Build history of the part. All positions in model axes, mm. A direction names the side the tool comes from. Coordinates: 2 decimals unless noted, no trailing zeros. Loops run counter-clockwise (first coordinate to the right, second up) from the corner with the lowest first, then second, coordinate; pieces in that order, holes last. Notation, with made-up numbers: (-12.5, 17) - (13.5, 17) arc R23 ccw to (13.5, 38) - close; hole circle Ø5 at (40, 2). An arc over 180 degrees is marked (long way). One line per item, written item: value.
```python
from build123d import *

# Parameters (mm, degrees)
BOTTOM_SECTION_BASE_SKETCH_W             = 15
BOTTOM_SECTION_BASE_SKETCH_H             = 15
BOTTOM_SECTION_EXTRUDE_DEPTH             = 40
HINGE_CUTOUT_SKETCH_W                    = 7
HINGE_CUTOUT_SKETCH_H                    = 15
HINGE_CUTOUT_EXTRUDED_CUT_DEPTH          = 15
HINGE_HOLE_SKETCH_R                      = 1
HINGE_HOLE_EXTRUDED_CUT_DEPTH            = 44.373378932
HINGER_CORNER_FILLETS_R                  = 5
STYLE_FILLETS_R                          = 1
ROUTING_HOLES_SKETCH_W                   = 2
ROUTING_HOLES_SKETCH_H                   = 2
ROUTING_HOLES_EXTRUDED_CUT_DEPTH         = 42.382363393
BACKING_START                            = -3.5
BACKING_EXTRUDE_DEPTH                    = 7
BOTTOM_SECTION_CONNECTION_HOLE_R         = 1.75
BOTTOM_SECTION_CONNECTION_HOLE_CUT_DEPTH = 3
SKETCH2_W                                = 7
SKETCH2_H                                = 2
BOTTOM_EXTENSION_EXTRUDE_DEPTH           = 6.5
FILLET1_R                                = 0.5


# Read off the part's stored shape, not the designer's step: Backing Extrude
with BuildPart() as part:
    # Bottom Section Base Sketch → Bottom Section Extrude (new body)
    with BuildSketch(Plane.XY):
        Rectangle(BOTTOM_SECTION_BASE_SKETCH_W, BOTTOM_SECTION_BASE_SKETCH_H)
    extrude(amount=BOTTOM_SECTION_EXTRUDE_DEPTH)

    # Hinge Cutout Sketch → Hinge Cutout Extruded Cut (cut)
    with BuildSketch(Plane.XY):
        Rectangle(HINGE_CUTOUT_SKETCH_W, HINGE_CUTOUT_SKETCH_H)
    hinge_cutout_extruded_cut = extrude(amount=HINGE_CUTOUT_EXTRUDED_CUT_DEPTH, mode=Mode.SUBTRACT)

    # Hinge Hole Sketch → Hinge Hole Extruded Cut (cut, through all)
    with BuildSketch(Plane(origin=(7.5, 0, 0), x_dir=(0, 0, -1), z_dir=(1, 0, 0))):
        with Locations((-5, 0)):
            Circle(HINGE_HOLE_SKETCH_R)
    hinge_hole_extruded_cut = extrude(amount=-HINGE_HOLE_EXTRUDED_CUT_DEPTH, mode=Mode.SUBTRACT)

    # Hinge and Hole Cutout Mirror: Hinge Cutout Extruded Cut, Hinge Hole Extruded Cut across plane
    add(hinge_cutout_extruded_cut.mirror(Plane.XY.offset(20)), mode=Mode.SUBTRACT)
    add(hinge_hole_extruded_cut.mirror(Plane.XY.offset(20)), mode=Mode.SUBTRACT)

    # Hinger Corner Fillets
    hinger_corner_fillets_edges = [part.edges().sort_by_distance(p)[0] for p in [
        (5.5, -7.5, 0),
        (-5.5, 7.5, 0),
        (-5.5, -7.5, 40),
        (-5.5, 7.5, 40),
        (5.5, -7.5, 40),
        (-5.5, -7.5, 0),
        (5.5, 7.5, 0),
        (5.5, 7.5, 40),
    ]]
    fillet(hinger_corner_fillets_edges, radius=HINGER_CORNER_FILLETS_R)

    # Style Fillets
    style_fillets_edges = [part.edges().sort_by_distance(p)[0] for p in [
        (7.5, 0, 40),
        (7.5, 7.5, 20),
        (-7.5, 7.5, 20),
        (7.5, 0, 0),
        (7.5, -7.5, 20),
        (7.5, 6.035533906, 1.464466094),
        (7.5, -6.035533906, 1.464466094),
        (7.5, -6.035533906, 38.535533906),
        (7.5, 6.035533906, 38.535533906),
        (-7.5, -7.5, 20),
        (-7.5, 0, 40),
        (-7.5, 0, 0),
        (-7.5, -6.035533906, 1.464466094),
        (-7.5, 6.035533906, 1.464466094),
        (-7.5, 6.035533906, 38.535533906),
        (-7.5, -6.035533906, 38.535533906),
    ]]
    fillet(style_fillets_edges, radius=STYLE_FILLETS_R)

    # Routing Holes Sketch → Routing Holes Extruded Cut (cut, through all)
    with BuildSketch(Plane.XY):
        with Locations((0, 4.5)):
            Rectangle(ROUTING_HOLES_SKETCH_W, ROUTING_HOLES_SKETCH_H)
        with Locations((0, -4.5)):
            Rectangle(ROUTING_HOLES_SKETCH_W, ROUTING_HOLES_SKETCH_H)
    extrude(amount=ROUTING_HOLES_EXTRUDED_CUT_DEPTH, mode=Mode.SUBTRACT)

    # Backing Extrude outline → Backing Extrude (add)
    with BuildSketch(Plane.YZ.offset(BACKING_START)):
        Polygon((-7.5, 32.145884327), (-7.5, 25), (-5.5, 25), (-5.5, 32.106829325), align=None)
    extrude(amount=BACKING_EXTRUDE_DEPTH)

    # Bottom Section Connection Hole → Bottom Section Connection Hole Cut (cut)
    with BuildSketch(Plane(origin=(7.5, 0, 0), x_dir=(0, 0, -1), z_dir=(1, 0, 0))):
        with Locations((-20, 0)):
            Circle(BOTTOM_SECTION_CONNECTION_HOLE_R)
    bottom_section_connection_hole_cut = extrude(amount=-BOTTOM_SECTION_CONNECTION_HOLE_CUT_DEPTH, mode=Mode.SUBTRACT)

    # Sketch2 → Bottom extension Extrude (add)
    with BuildSketch(Plane(origin=(0, 0, 15), x_dir=(-1, 0, 0), z_dir=(0, 0, -1))):
        with Locations((0, -6.5)):
            Rectangle(SKETCH2_W, SKETCH2_H)
    extrude(amount=BOTTOM_EXTENSION_EXTRUDE_DEPTH)

    # Connection Hole Mirror: Bottom Section Connection Hole Cut across plane
    add(bottom_section_connection_hole_cut.mirror(Plane(origin=(0, 0, 0), x_dir=(0, 0, 1), z_dir=(1, 0, 0))), mode=Mode.SUBTRACT)

    # Fillet1
    fillet1_edges = [part.edges().sort_by_distance(p)[0] for p in [
        (-1, -4.5, 25),
        (0, -3.5, 25),
        (1, -4.5, 25),
        (0, 5.5, 25),
        (1, 4.5, 25),
        (0, 3.5, 25),
        (-1, 4.5, 25),
        (-1, 4.5, 15),
        (0, 3.5, 15),
        (1, 4.5, 15),
        (0, 5.5, 15),
        (1, -4.5, 15),
        (0, -3.5, 15),
        (-1, -4.5, 15),
    ]]
    fillet(fillet1_edges, radius=FILLET1_R)


solid = part.part
```
Item 1: Cut at C-C, the plane x = 6. Write the cut outline in (y, z).
Check result:
outline: (-7.5, 5) arc R5 ccw to (-2.5, 0) - (2.5, 0) arc R5 ccw to (7.5, 5) - (7.5, 35) arc R5 ccw to (2.5, 40) - (-2.5, 40) arc R5 ccw to (-7.5, 35) - close; hole circle Ø3.5 at (0, 20); hole circle Ø2 at (0, 5); hole circle Ø2 at (0, 35)
Item 2: Probe probe 1 along X at (y, z) = (5.75, 36); probe 2 along Y at (x, z) = (-6, 5); probe 3 along Z at (x, y) = (1.25, -0.5). List the from-to ranges inside material, lowest first. Write a range as from..to.
Check result:
probe 1: x = -7.5..-3.5, 3.5..7.5
probe 2: y = -7.5..-1, 1..7.5
probe 3: z = 15..25
Item 3: Cut at A-A, the plane z = 33. Write the cut outline in (x, y).
Check result:
outline: (-7.5, -6.5) arc R1 ccw to (-6.5, -7.5) - (-3.5, -7.5) - (-3.5, 7.5) - (-6.5, 7.5) arc R1 ccw to (-7.5, 6.5) - close; (3.5, -7.5) - (6.5, -7.5) arc R1 ccw to (7.5, -6.5) - (7.5, 6.5) arc R1 ccw to (6.5, 7.5) - (3.5, 7.5) - close
Item 4: Tool access for faces 4 (the face through (-3.5, 0, 33)), 5 (the face through (1, 4, 20)), 6 (the face through (0, -6, 8.5)): list every direction of +Z, -Z, +X, -X, +Y, -Y with a clear straight run to the whole face (end or side of a thin tool).
Check result:
face 4: +Z, +Y
face 5: +Z, -Z
face 6: -Z, +Y, -Y
Item 5: Pull direction X, two halves, no side cores. Call faces 1 (the face through (6.02, 0.08, 21.75)), 2 (the face through (-3.5, 0, 7)), 3 (the face through (7.215, -7.199, 20.21)): released by +X, released by -X, zero draft, split by the parting line, or undercut.
Check result:
face 1: zero draft
face 2: undercut
face 3: released by +X
Item 6: Cut at D-D, the plane z = 20. Write the cut outline in (x, y).
Check result:
outline: (-7.5, -6.5) arc R1 ccw to (-6.5, -7.5) - (6.5, -7.5) arc R1 ccw to (7.5, -6.5) - (7.5, -1.75) - (4.5, -1.75) - (4.5, 1.75) - (7.5, 1.75) - (7.5, 6.5) arc R1 ccw to (6.5, 7.5) - (-6.5, 7.5) arc R1 ccw to (-7.5, 6.5) - (-7.5, 1.75) - (-4.5, 1.75) - (-4.5, -1.75) - (-7.5, -1.75) - close; hole (-1, -5.5) - (1, -5.5) - (1, -3.5) - (-1, -3.5) - close; hole (-1, 3.5) - (1, 3.5) - (1, 5.5) - (-1, 5.5) - close
Item 7: Cut at B-B, the plane x = 0.5. Write the cut outline in (y, z).
Check result:
outline: (-7.5, 8.5) - (-5.5, 8.5) - (-5.5, 32.11) - (-7.5, 32.15) - close; (-3.5, 15.5) arc R0.5 ccw to (-3, 15) - (3, 15) arc R0.5 ccw to (3.5, 15.5) - (3.5, 24.5) arc R0.5 ccw to (3, 25) - (-3, 25) arc R0.5 ccw to (-3.5, 24.5) - close; (5.5, 15.5) arc R0.5 ccw to (6, 15) - (7.5, 15) - (7.5, 25) - (6, 25) arc R0.5 ccw to (5.5, 24.5) - close
Item 8: Drop flat-ended pins along their axis: P1, Ø1, axis at y = 0, z = 20.5, coming from the -X side; P2, Ø2, axis at x = 0.5, y = -7, coming from the -Z side. Give the stop position or say it passes through.
Check result:
P1: stops at x = -4.5
P2: stops at z = 8.5
